Part model, mm, in its own coordinate system. Face numbers are marked on the shaded views. A direction names the side the tool comes from. Coordinates: 2 decimals unless noted, no trailing zeros. Loops run counter-clockwise (first coordinate to the right, second up) from the corner with the lowest first, then second, coordinate; pieces in that order, holes last. Notation, with made-up numbers: (19.5, 66) -> (61.5, 66) arc R10 cw to (61.5, 84) -> close; hole circle Ø9 at (7, 11). An arc over 180 degrees is marked (long way). Use one line per item in the form item = value. Start each with the question number.
(1) Mould opens along X. For the marked faces 4, 5, 6 and 7 say: +X half, -X half, draft (parallel to the pull), parting line (faces both ways), or undercut.
(2) Band-saw the part on C-C on y = 176. Give the cut face in (x, z), then the cut area to 3 significant figures.
(3) 3-axis set-ups, long thin cutter, end or side, ignore diameter. For the marked faces 1, 2 and 3: which of +Z, -Z, +X, -X, +Y, -Y reach the whole face in a straight line?
(4) Drill centre lines: L1, parallel to Y at x = 73, z = 36.5; L2, parallel to Y at x = 0, z = 12; L3, parallel to Y at x = 0, z = 32. Where is each one in solid material? Low to high. Write a range as [from, to].
(5) Pin check, flat tips, straight feed: P1, Ø3, axis at x = -31, z = 23, coming from the +Y side (3 decimals); P2, Ø8, axis at x = 59.5, z = 42, coming from the +Y side; P3, Ø2, axis at y = -110, z = 36, coming from the +X side. Stop position of each tip, or through.
(6) Band-saw the part on D-D on z = 16.5. Give the cut face in (x, y), then the cut area to 3 significant figures.
(7) Band-saw the part on A-A on z = 37. Give the cut face in (x, y).
(8) Band-saw the part on B-B on x = 0. Give the cut face in (y, z), then the cut area to 3 significant figures.
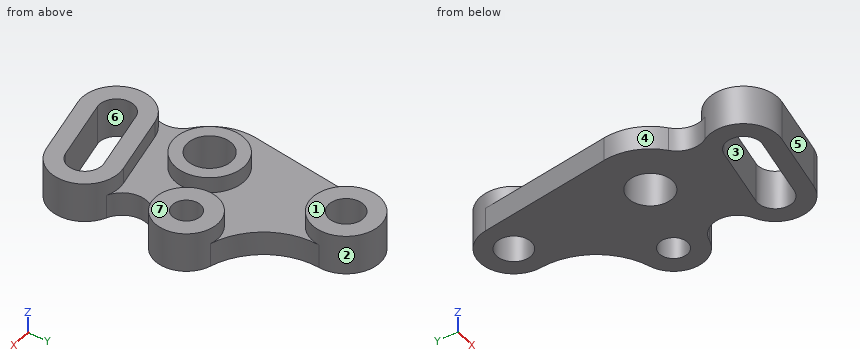
```python
from build123d import *

# Parameters (mm, degrees)
SKETCH1_R           = 44
BOSS_EXTRUDE1_DEPTH = 30
SKETCH1_3_R         = 43
SKETCH1_3_R_2       = 22
SKETCH1_3_R_3       = 40
SKETCH1_3_R_4       = 18
SKETCH1_3_R_5       = 44
SKETCH1_3_R_6       = 28
BOSS_EXTRUDE2_DEPTH = 50


with BuildPart() as part:
    # Sketch1 → Boss-Extrude1 (new body)
    with BuildSketch(Plane.XY):
        with BuildLine():
            ThreePointArc((-37.152695317, -96.427192982), (-25.310496196, -84.008629057), (-9.618664602, -77.064218986))
            Line((-9.618664602, -77.064218986), (75.140384229, -58.076119936))
            ThreePointArc((75.140384229, -58.076119936), (88.978408325, -57.214674948), (102.397475744, -60.702027518))
            ThreePointArc((102.397475744, -60.702027518), (83.306238653, -29.112938991), (106.680790328, -0.547642184))
            ThreePointArc((106.680790328, -0.547642184), (56, 38), (106.680790328, 76.547642184))
            ThreePointArc((106.680790328, 76.547642184), (57.263244705, 112.084196354), (42.730356863, 171.192027211))
            ThreePointArc((42.730356863, 171.192027211), (-5.703537617, 133.379938308), (-42.49099891, 182.596590909))
            Line((-42.49099891, 182.596590909), (-69.171393575, 10.738636364))
            ThreePointArc((-69.171393575, 10.738636364), (-65.309307933, -25.193139885), (-44.040182506, -54.410130719))
            ThreePointArc((-44.040182506, -54.410130719), (-32.594285398, -74.106939259), (-37.152695317, -96.427192982))
        make_face()
        Circle(SKETCH1_R, mode=Mode.SUBTRACT)
    extrude(amount=BOSS_EXTRUDE1_DEPTH)

    # Sketch1_3 → Boss-Extrude2 (add)
    # profile 1 of 4: a face of its own
    with BuildSketch(Plane.XY):
        with Locations(Location((0, 176, 0), (0, 0, 171.175459611))):
            Circle(SKETCH1_3_R)
        with Locations((0, 176)):
            Circle(SKETCH1_3_R_2, mode=Mode.SUBTRACT)
    # profile 2 of 4: a face of its own
    with BuildSketch(Plane.XY):
        with Locations(Location((96, 38, 0), (0, 0, 285.487001772))):
            Circle(SKETCH1_3_R_3)
        with Locations((96, 38)):
            Circle(SKETCH1_3_R_4, mode=Mode.SUBTRACT)
    # profile 3 of 4: a face of its own
    with BuildSketch(Plane.XY):
        Circle(SKETCH1_3_R_5)
        Circle(SKETCH1_3_R_6, mode=Mode.SUBTRACT)
    # profile 4 of 4: a face of its own
    with BuildSketch(Plane.XY):
        with BuildLine():
            Line((9.618664602, -162.935781014), (94.377713433, -143.947681963))
            ThreePointArc((94.377713433, -143.947681963), (127.694829845, -91.393236347), (75.140384229, -58.076119936))
            Line((75.140384229, -58.076119936), (-9.618664602, -77.064218986))
            ThreePointArc((-9.618664602, -77.064218986), (-42.935781014, -129.618664602), (9.618664602, -162.935781014))
        make_face()
        with BuildLine():
            ThreePointArc((-4.809332301, -98.532109493), (-21.467890507, -124.809332301), (4.809332301, -141.467890507))
            Line((4.809332301, -141.467890507), (89.568381132, -122.479791457))
            ThreePointArc((89.568381132, -122.479791457), (106.226939338, -96.202568649), (79.94971653, -79.544010443))
            Line((79.94971653, -79.544010443), (-4.809332301, -98.532109493))
        make_face(mode=Mode.SUBTRACT)
    extrude(amount=BOSS_EXTRUDE2_DEPTH)


solid = part.part
```
A:
q1.face_4 = -X half
q1.face_5 = +X half
q1.face_6 = undercut
q1.face_7 = draft
q2.outline = (-43.52, 0) -> (-22, 0) -> (-22, 50) -> (-43, 50) -> (-43, 30) -> (-43.52, 30) -> close; (22, 0) -> (43, 0) -> (43, 50) -> (22, 50) -> close
q2.area = 2,120 mm²
q3.face_1 = +Z, +X, -X, +Y, -Y
q3.face_2 = +Z
q3.face_3 = +Z, -Z
q4.L1 = [-148.74, -126.19], [-81.1, -58.56], [5.27, 70.73]
q4.L2 = [-164, -142], [-97.45, -28], [28, 154], [198, 219]
q4.L3 = [-164, -142], [-97.45, -74.91], [-44, -28], [28, 44], [133, 154], [198, 219]
q5.P1 = 207.285
q5.P2 = 61.32
q5.P3 = 128.03
q6.outline = (-69.17, 10.74) arc R70 ccw to (-44.04, -54.41) arc R32 cw to (-37.15, -96.43) arc R44 ccw to (9.62, -162.94) -> (94.38, -143.95) arc R44 ccw to (102.4, -60.7) arc R32 cw to (106.68, -0.55) arc R40 ccw to (106.68, 76.55) arc R88 cw to (42.73, 171.19) arc R43 ccw to (-42.49, 182.6) -> close; hole circle Ø56 at (0, 0); hole circle Ø44 at (0, 176); hole (-4.81, -98.53) arc R22 ccw to (4.81, -141.47) -> (89.57, -122.48) arc R22 ccw to (79.95, -79.54) -> close; hole circle Ø36 at (96, 38)
q6.area = 41,900 mm²
q7.outline = circle Ø88 at (0, 0); circle Ø86 at (0, 176); (-9.62, -77.06) arc R44 ccw to (9.62, -162.94) -> (94.38, -143.95) arc R44 ccw to (75.14, -58.08) -> close; circle Ø80 at (96, 38); hole circle Ø56 at (0, 0); hole circle Ø44 at (0, 176); hole (-4.81, -98.53) arc R22 ccw to (4.81, -141.47) -> (89.57, -122.48) arc R22 ccw to (79.95, -79.54) -> close; hole circle Ø36 at (96, 38)
q8.outline = (-164, 0) -> (-142, 0) -> (-142, 50) -> (-164, 50) -> close; (-97.45, 0) -> (-28, 0) -> (-28, 50) -> (-44, 50) -> (-44, 30) -> (-74.91, 30) -> (-74.91, 50) -> (-97.45, 50) -> close; (28, 0) -> (154, 0) -> (154, 50) -> (133, 50) -> (133, 30) -> (44, 30) -> (44, 50) -> (28, 50) -> close; (198, 0) -> (219, 0) -> (219, 50) -> (198, 50) -> close
q8.area = 9,520 mm²
